Geometry check sheet. Reference: drawing and pictorial views, mm from the part's lowest x, y, z. A direction names the side the tool comes from. Round coordinates to 2 decimals unless told otherwise and drop trailing zeros. Order: outer loops, then holes, each group sorted by start corner. A loop starts at its lowest first (then second) coordinate and runs counter-clockwise, first axis right, second up.
(1) Go/stop test with flat-tipped pins: pin 1 (12 mm diameter, centred on y = 10, z = 7.5, fed in from -X); pin 2 (7.5 mm diameter, centred on y = 20.5, z = 5.72, fed in from +X); pin 3 (3 mm diameter, centred on x = 18, z = 8, fed in from +Y). Record where each tip stops, or that it passes through.
(2) Sectioned sample at C-C (z = 35.5). Record the boundary of the cut face in (x, y).
(3) Sectioned sample at B-B (y = 34). Record the boundary of the cut face in (x, z).
(4) Sectioned sample at A-A (x = 35.5). Record the boundary of the cut face in (y, z), plus the area to 3 significant figures.
(5) Material ranges on line 1 along X through (y, z) = (3.75, 32); line 2 along Y through (x, z) = (7, 20); line 3 along Y through (x, z) = (11.5, 10), recorded low to high.
(6) Sectioned sample at D-D (x = 18). Record the boundary of the cut face in (y, z).
(7) Release check for a two-part mould opening along Y. For the marked faces 3, 4 and 5 record: +Y half, -Y half, draft (parallel to the pull), parting line (faces both ways), or undercut.
(8) Set-up check for the marked faces 1 and 2: record each of +Z, -Z, +X, -X, +Y, -Y from which the full face is reachable in a straight line by a thin tool's end or side.
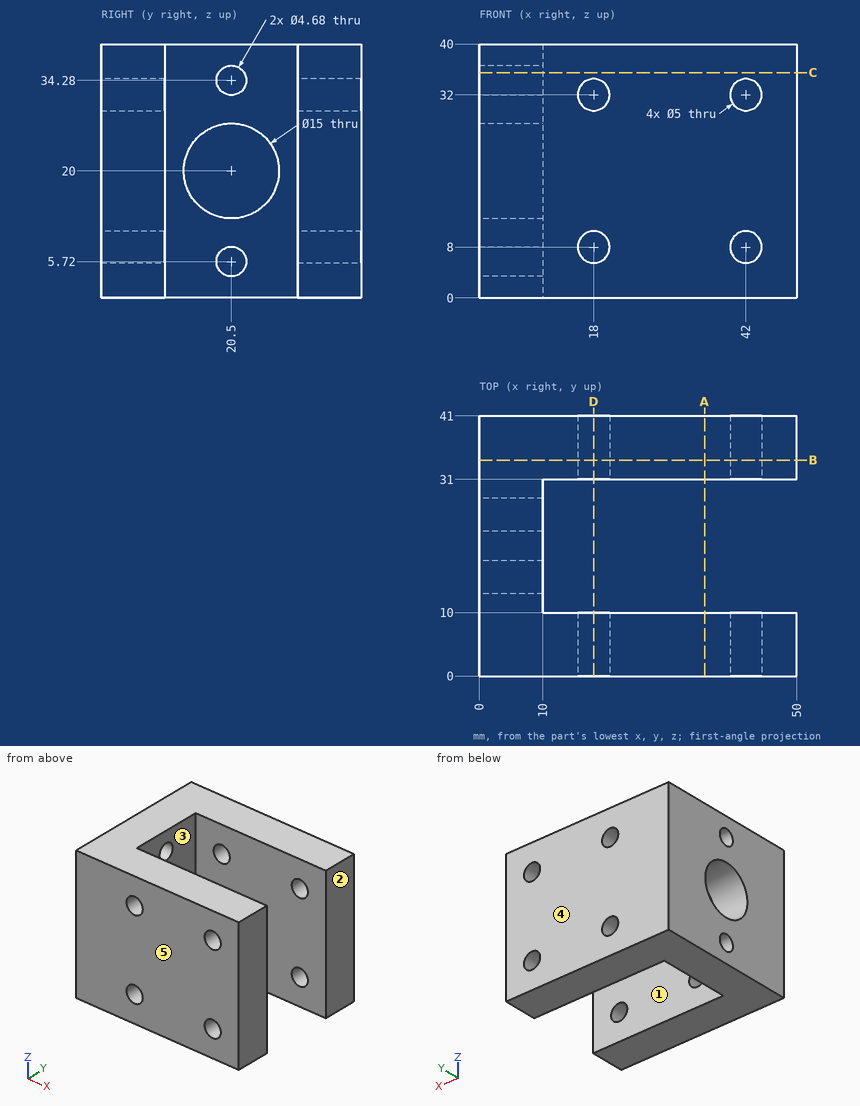
Answer below:
1. pin 1: stops at x = 0
1. pin 2: stops at x = 10
1. pin 3: passes through
2. outline: (0, 0) - (50, 0) - (50, 10) - (10, 10) - (10, 18.5) - (0, 18.5) - close; (0, 22.5) - (10, 22.5) - (10, 31) - (50, 31) - (50, 41) - (0, 41) - close
3. outline: (0, 0) - (50, 0) - (50, 40) - (0, 40) - close; hole circle Ø5 at (18, 8); hole circle Ø5 at (18, 32); hole circle Ø5 at (42, 8); hole circle Ø5 at (42, 32)
4. outline: (0, 0) - (10, 0) - (10, 40) - (0, 40) - close; (31, 0) - (41, 0) - (41, 40) - (31, 40) - close
4. area: 800 mm2
5. line 1: x = 0 to 15.5, 20.5 to 39.5, 44.5 to 50
5. line 2: y = 0 to 13, 28 to 41
5. line 3: y = 0 to 10, 31 to 41
6. outline: (0, 0) - (10, 0) - (10, 5.5) - (0, 5.5) - close; (0, 10.5) - (10, 10.5) - (10, 29.5) - (0, 29.5) - close; (0, 34.5) - (10, 34.5) - (10, 40) - (0, 40) - close; (31, 0) - (41, 0) - (41, 5.5) - (31, 5.5) - close; (31, 10.5) - (41, 10.5) - (41, 29.5) - (31, 29.5) - close; (31, 34.5) - (41, 34.5) - (41, 40) - (31, 40) - close
7. face 3: undercut
7. face 4: +Y half
7. face 5: -Y half
8. face 1: +Z, -Z, +X
8. face 2: +Z, -Z, +X, +Y, -Y
